CAD build for the part. Positions are in the model's coordinates, mm. A direction names the side the tool comes from. Round coordinates to 2 decimals unless told otherwise and drop trailing zeros. Write each loop counter-clockwise with the first axis right and the second up, starting at its lowest first coordinate (ties: lowest second). Pieces come first, ordered by that corner, then holes. Notation, with made-up numbers: (54, 0.5) - (63, 0.5) arc R12 ccw to (63, 9.5) - close; hole circle Ø1 at (-34.75, -28.75). An arc over 180 degrees is marked (long way). Put each result on its own line as item: value. Start each with the question number.
Item 1: Pin check, flat tips, straight feed: pin 1 Ø3 at (y, z) = (-14, 0) entering from +X; pin 2 Ø6.5 at (y, z) = (-15.5, 1) entering from -X. Stop position of each tip, or through.
Item 2: Cut at D-D (z = 5). Give the cut face in (x, y), and give its area (3 significant figures).
Item 3: Mould opens along X. For faces 6 (the flat face through (-56.833, -11, 17)), 7 (the flat face through (-44.16, -11.27, 0.03)), 8 (the flat face through (-51, -11, -12.526)) say: released by +X, released by -X, zero draft, split by the parting line, or undercut.
Item 4: Cut at B-B (z = -7). Give the cut face in (x, y).
Item 5: 3-axis set-ups, long thin cutter, end or side, ignore diameter. For faces 1 (the flat face through (-44.248, -11, -10)), 2 (the flat face through (-21, -11, 14.203)), 3 (the flat face through (-18.993, -11, 17)), 4 (the flat face through (-55, -11, -8.48)), 5 (the flat face through (-32.24, -11.27, -0.03)): which of +Z, -Z, +X, -X, +Y, -Y reach the whole face in a straight line?
Item 6: Drill centre lines: line 1 (X direction, y = -6, z = 6.5); line 2 (Z direction, x = -20.5, y = -11.25); line 3 (X direction, y = -20.75, z = -6). Where is each one in solid material? Low to high. Write a range as from..to.
Item 7: Cut at A-A (x = -21.5). Give the cut face in (y, z), and give its area (3 significant figures).
Item 8: Cut at C-C (y = -21.5). Give the cut face in (x, z), and give its area (3 significant figures).
```python
from build123d import *

# Parameters (mm, degrees)
F0_R     = 0.54548
F1_DEPTH = 22.86


with BuildPart() as f1:
    # F0 (on Front) → F1 (new body)
    with BuildSketch(Plane.XZ):
        Polygon((-31.546149, -12.525664), (-18.993298, -12.525664), (-18.993298, -8.878619), (-20.582533, -8.872862), (-22.865418, -8.872862), (-22.865418, 14.203154), (-20.582533, 14.203154), (-18.993298, 14.203154), (-18.993298, 18.924711), (-31.999168, 18.924711), (-38.48568, -2.924589), (-44.079449, 18.924711), (-56.833036, 18.924711), (-56.833036, 14.379703), (-53.468131, 14.379703), (-53.468131, -8.480297), (-56.833036, -8.480297), (-56.833036, -12.525664), (-44.248171, -12.525664), (-44.248171, -8.242098), (-47.813166, -8.242098), (-47.813166, 12.242473), (-40.400241, -12.525664), (-35.947602, -12.525664), (-28.42512, 12.813221), (-28.42512, -8.844449), (-31.546149, -8.844449), align=None)
        with Locations((-55.57109, 17.791551)):
            Circle(F0_R, mode=Mode.SUBTRACT)
    extrude(amount=F1_DEPTH)


solid = f1.part
```
Output values:
1. pin 1: x = -22.87
1. pin 2: x = -53.47
2. outline: (-53.47, -22.86) - (-47.81, -22.86) - (-47.81, 0) - (-53.47, 0) - close; (-45.65, -22.86) - (-40.51, -22.86) - (-40.51, 0) - (-45.65, 0) - close; (-36.13, -22.86) - (-30.74, -22.86) - (-30.74, 0) - (-36.13, 0) - close; (-28.43, -22.86) - (-22.87, -22.86) - (-22.87, 0) - (-28.43, 0) - close
2. area: 497 mm2
3. face 6: released by -X
3. face 7: undercut
3. face 8: zero draft
4. outline: (-53.47, -22.86) - (-47.81, -22.86) - (-47.81, 0) - (-53.47, 0) - close; (-42.05, -22.86) - (-34.31, -22.86) - (-34.31, 0) - (-42.05, 0) - close; (-28.43, -22.86) - (-22.87, -22.86) - (-22.87, 0) - (-28.43, 0) - close
5. face 1: -Z, +Y, -Y
5. face 2: +X, +Y, -Y
5. face 3: +Z, -Z, +X, +Y, -Y
5. face 4: -X, +Y, -Y
5. face 5: +Y, -Y
6. line 1: -53.47..-47.81, -46.09..-40.9, -35.69..-30.3, -28.43..-22.87
6. line 2: -12.53..-8.87, 14.2..18.92
6. line 3: -53.47..-47.81, -42.35..-34.01, -28.43..-22.87
7. outline: (-22.86, -12.53) - (0, -12.53) - (0, -8.87) - (-22.86, -8.87) - close; (-22.86, 14.2) - (0, 14.2) - (0, 18.92) - (-22.86, 18.92) - close
7. area: 191 mm2
8. outline: (-56.83, -12.53) - (-44.25, -12.53) - (-44.25, -8.24) - (-47.81, -8.24) - (-47.81, 12.24) - (-40.4, -12.53) - (-35.95, -12.53) - (-28.43, 12.81) - (-28.43, -8.84) - (-31.55, -8.84) - (-31.55, -12.53) - (-18.99, -12.53) - (-18.99, -8.88) - (-20.58, -8.87) - (-22.87, -8.87) - (-22.87, 14.2) - (-18.99, 14.2) - (-18.99, 18.92) - (-32, 18.92) - (-38.49, -2.92) - (-44.08, 18.92) - (-56.83, 18.92) - (-56.83, 14.38) - (-53.47, 14.38) - (-53.47, -8.48) - (-56.83, -8.48) - close; hole circle Ø1.09 at (-55.57, 17.79)
8. area: 731 mm2
